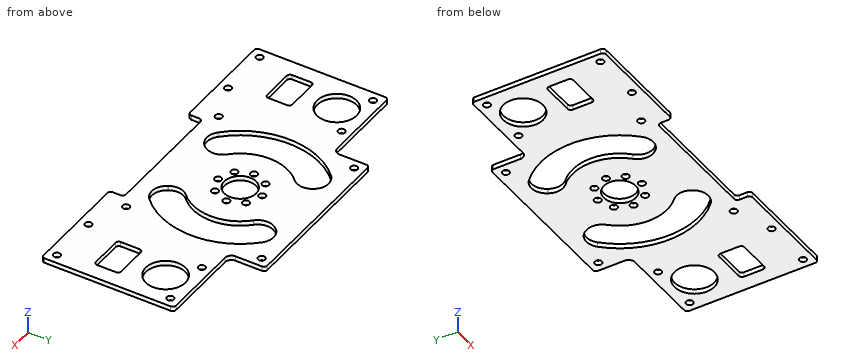
```python
from build123d import *

# Parameters (mm, degrees)
F0_W     = 109
F0_H     = 70
F0_R     = 1.1
F0_R_2   = 6.3
F1_DEPTH = 1.5
F2_R     = 5.05
F2_R_2   = 1.1
F2_W     = 53
F2_H     = 10.5
F2_W_2   = 40
F2_H_2   = 10.5680569839
F3_DEPTH = 1.5
F4_W     = 34.5
F4_H     = 6
F5_DEPTH = 1.5
F6_R     = 1


with BuildPart() as f1:
    # F0 (on Top) → F1 (new body)
    with BuildSketch(Plane.XY):
        Rectangle(F0_W, F0_H)
        with Locations((-51.5, -26)):
            Circle(F0_R, mode=Mode.SUBTRACT)
        with Locations((-35.5, -26)):
            Circle(F0_R, mode=Mode.SUBTRACT)
        with Locations((-23.5, -21.5)):
            Circle(F0_R, mode=Mode.SUBTRACT)
        with BuildLine():
            ThreePointArc((-37.5, -14.5), (-37.7928932188, -15.2071067812), (-38.5, -15.5))
            Line((-38.5, -15.5), (-48.5, -15.5))
            ThreePointArc((-48.5, -15.5), (-49.2071067812, -15.2071067812), (-49.5, -14.5))
            Line((-49.5, -14.5), (-49.5, -8.5))
            ThreePointArc((-49.5, -8.5), (-49.2071067812, -7.7928932188), (-48.5, -7.5))
            Line((-48.5, -7.5), (-38.5, -7.5))
            ThreePointArc((-38.5, -7.5), (-37.7928932188, -7.7928932188), (-37.5, -8.5))
            Line((-37.5, -8.5), (-37.5, -14.5))
        make_face(mode=Mode.SUBTRACT)
        with Locations((23.5, -21.5)):
            Circle(F0_R, mode=Mode.SUBTRACT)
        with Locations((35.5, -26)):
            Circle(F0_R, mode=Mode.SUBTRACT)
        with Locations((51.5, -26)):
            Circle(F0_R, mode=Mode.SUBTRACT)
        with BuildLine():
            Line((38.5, -7.5), (48.5, -7.5))
            ThreePointArc((48.5, -7.5), (49.2071067812, -7.7928932188), (49.5, -8.5))
            Line((49.5, -8.5), (49.5, -14.5))
            ThreePointArc((49.5, -14.5), (49.2071067812, -15.2071067812), (48.5, -15.5))
            Line((48.5, -15.5), (38.5, -15.5))
            ThreePointArc((38.5, -15.5), (37.7928932188, -15.2071067812), (37.5, -14.5))
            Line((37.5, -14.5), (37.5, -8.5))
            ThreePointArc((37.5, -8.5), (37.7928932188, -7.7928932188), (38.5, -7.5))
        make_face(mode=Mode.SUBTRACT)
        with Locations((-43.5, 3.5)):
            Circle(F0_R_2, mode=Mode.SUBTRACT)
        with Locations((-51.5, 10)):
            Circle(F0_R, mode=Mode.SUBTRACT)
        with Locations((-35.5, 10)):
            Circle(F0_R, mode=Mode.SUBTRACT)
        with Locations((-23.5, 21.5)):
            Circle(F0_R, mode=Mode.SUBTRACT)
        with Locations((43.5, 3.5)):
            Circle(F0_R_2, mode=Mode.SUBTRACT)
        with Locations((35.5, 10)):
            Circle(F0_R, mode=Mode.SUBTRACT)
        with Locations((51.5, 10)):
            Circle(F0_R, mode=Mode.SUBTRACT)
        with Locations((23.5, 21.5)):
            Circle(F0_R, mode=Mode.SUBTRACT)
    extrude(amount=F1_DEPTH)

    # F2 (on face) → F3 (cut, through all)
    with BuildSketch(Plane.XY.offset(1.5)):
        Circle(F2_R)
        with Locations((0, 7)):
            Circle(F2_R_2)
        with Locations((-4.9497474683, 4.9497474683)):
            Circle(F2_R_2)
        with Locations((-7, 0)):
            Circle(F2_R_2)
        with Locations((-4.9497474683, -4.9497474683)):
            Circle(F2_R_2)
        with Locations((0, -7)):
            Circle(F2_R_2)
        with Locations((4.9497474683, -4.9497474683)):
            Circle(F2_R_2)
        with Locations((7, 0)):
            Circle(F2_R_2)
        with Locations((4.9497474683, 4.9497474683)):
            Circle(F2_R_2)
        with BuildLine():
            ThreePointArc((-9.7467943448, 16.8819430161), (-13.3130208521, 19.2849078273), (-17.4008940589, 17.9501778808))
            ThreePointArc((-17.4008940589, 17.9501778808), (-25, 0), (-17.4008940589, -17.9501778808))
            ThreePointArc((-17.4008940589, -17.9501778808), (-13.3130208521, -19.2849078273), (-9.7467943448, -16.8819430161))
            Line((-9.7467943448, -16.8819430161), (-9.643650761, -16.7032930885))
            ThreePointArc((-9.643650761, -16.7032930885), (-9.0333585083, -13.5821275803), (-10.4677200298, -10.7436882577))
            ThreePointArc((-10.4677200298, -10.7436882577), (-15, 0), (-10.4677200298, 10.7436882577))
            ThreePointArc((-10.4677200298, 10.7436882577), (-9.0333585083, 13.5821275803), (-9.643650761, 16.7032930885))
            Line((-9.643650761, 16.7032930885), (-9.7467943448, 16.8819430161))
        make_face()
        with BuildLine():
            ThreePointArc((17.4008940589, 17.9501778808), (13.3130208521, 19.2849078273), (9.7467943448, 16.8819430161))
            Line((9.7467943448, 16.8819430161), (9.643650761, 16.7032930885))
            ThreePointArc((9.643650761, 16.7032930885), (9.0333585083, 13.5821275803), (10.4677200298, 10.7436882577))
            ThreePointArc((10.4677200298, 10.7436882577), (15, 0), (10.4677200298, -10.7436882577))
            ThreePointArc((10.4677200298, -10.7436882577), (9.0333585083, -13.5821275803), (9.643650761, -16.7032930885))
            Line((9.643650761, -16.7032930885), (9.7467943448, -16.8819430161))
            ThreePointArc((9.7467943448, -16.8819430161), (13.3130208521, -19.2849078273), (17.4008940589, -17.9501778808))
            ThreePointArc((17.4008940589, -17.9501778808), (25, 0), (17.4008940589, 17.9501778808))
        make_face()
        with BuildLine():
            Line((-26.5, 35), (-54.5, 35))
            Line((-54.5, 35), (-54.5, 13))
            Line((-54.5, 13), (-28.5, 13))
            ThreePointArc((-28.5, 13), (-27.0857864376, 13.5857864376), (-26.5, 15))
            Line((-26.5, 15), (-26.5, 24.5))
            Line((-26.5, 24.5), (-26.5, 35))
        make_face()
        with Locations((0, 29.75)):
            Rectangle(F2_W, F2_H)
        with BuildLine():
            Line((54.5, 35), (26.5, 35))
            Line((26.5, 35), (26.5, 24.5))
            Line((26.5, 24.5), (26.5, 15))
            ThreePointArc((26.5, 15), (27.0857864376, 13.5857864376), (28.5, 13))
            Line((28.5, 13), (54.5, 13))
            Line((54.5, 13), (54.5, 35))
        make_face()
        with Locations((0, -29.7159715081)):
            Rectangle(F2_W_2, F2_H_2)
    extrude(amount=-F3_DEPTH, mode=Mode.SUBTRACT)

    # F4 (on face) → F5 (cut, through all)
    with BuildSketch(Plane.XY.offset(1.5)):
        with Locations((-37.25, -32)):
            Rectangle(F4_W, F4_H)
        with Locations((37.25, -32)):
            Rectangle(F4_W, F4_H)
    extrude(amount=-F5_DEPTH, mode=Mode.SUBTRACT)

    # F6
    f6_edges = [f1.edges().sort_by_distance(p)[0] for p in [
        (-54.5, -29, 0.75),
        (-20, -29, 0.75),
        (20, -29, 0.75),
        (54.5, -29, 0.75),
        (-20, -24.431943, 0.75),
        (20, -24.431943, 0.75),
        (54.5, 13, 0.75),
        (26.5, 24.5, 0.75),
        (-26.5, 24.5, 0.75),
        (-54.5, 13, 0.75),
    ]]
    fillet(f6_edges, radius=F6_R)


solid = f1.part
```
CAD build for the part. Positions are in the model's coordinates, mm. Round coordinates to 2 decimals unless told otherwise and drop trailing zeros. Order: outer loops, then holes, each group sorted by start corner. A loop starts at its lowest first (then second) coordinate and runs counter-clockwise, first axis right, second up.
Item 1: Probe line 1 along Y through (x, z) = (-35.5, 0.75); line 2 along Y through (x, z) = (-43.5, 1.1); line 3 along Y through (x, z) = (0, 0.5). List the from-to ranges inside material, lowest first.
Item 2: Saw through at D-D on z = 0.65. State how many separate pieces and enclosed holes the cut face has, then the cut area to 3 significant figures.
Item 3: Saw through at C-C on x = -23.5. Write the cut outline in (y, z).
Item 4: Pin check, flat tips, straight feed: pin 1 (0.8 mm diameter, centred on x = -8, z = 0.5, fed in from -Y); pin 2 (0.8 mm diameter, centred on x = 47, z = 1, fed in from +Y). Stop position of each tip, or through.
Item 5: Saw through at B-B on x = 51.5. Write the cut outline in (y, z), then the cut area to 3 significant figures.
Item 6: Saw through at A-A on y = 21.5. Write the cut outline in (x, z).
Reported:
1. line 1: y = -29 to -27.1, -24.9 to 8.9, 11.1 to 13
1. line 2: y = -29 to -15.5, -7.5 to -2.8, 9.8 to 13
1. line 3: y = -24.43 to -8.1, -5.9 to -5.05, 5.05 to 5.9, 8.1 to 24.5
2. separate pieces: 1
2. enclosed holes: 27
2. area: 3,610 mm2
3. outline: (-29, 0) - (-22.6, 0) - (-22.6, 1.5) - (-29, 1.5) - close; (-20.4, 0) - (-8.53, 0) - (-8.53, 1.5) - (-20.4, 1.5) - close; (8.53, 0) - (20.4, 0) - (20.4, 1.5) - (8.53, 1.5) - close; (22.6, 0) - (24.5, 0) - (24.5, 1.5) - (22.6, 1.5) - close
4. pin 1: stops at y = -24.43
4. pin 2: stops at y = 13
5. outline: (-29, 0) - (-27.1, 0) - (-27.1, 1.5) - (-29, 1.5) - close; (-24.9, 0) - (8.9, 0) - (8.9, 1.5) - (-24.9, 1.5) - close; (11.1, 0) - (13, 0) - (13, 1.5) - (11.1, 1.5) - close
5. area: 56.4 mm2
6. outline: (-26.5, 0) - (-24.6, 0) - (-24.6, 1.5) - (-26.5, 1.5) - close; (-22.4, 0) - (22.4, 0) - (22.4, 1.5) - (-22.4, 1.5) - close; (24.6, 0) - (26.5, 0) - (26.5, 1.5) - (24.6, 1.5) - close
